Check sheet for the modelled part. Datum: model origin and axes. Units: mm. A direction names the side the tool comes from. Round coordinates to 2 decimals unless told otherwise and drop trailing zeros. Order: outer loops, then holes, each group sorted by start corner. A loop starts at its lowest first (then second) coordinate and runs counter-clockwise, first axis right, second up. Notation, with made-up numbers: (-2.75, -14.5) -> (25.25, -14.5) arc R18 ccw to (25.25, 20.5) -> close; hole circle Ø10 at (43.25, 67.5). An arc over 180 degrees is marked (long way). Answer in a Markdown table with one row per item. Add a question column.
1. Draft check along X on faces 3 (the flat face through (0, -2.8, 7)), 4 (the flat face through (0, -4.5, 7)), 5 (the cylindrical face through (-8.115, 4.199, 6.987)). Enter one of: +X half, -X half, draft (parallel to the pull), parting line (faces both ways), or undercut.
2. Sectioned sample at A-A, the plane x = -2.75. Record the boundary of the cut face in (y, z), then the cut area to 3 significant figures.
3. Sectioned sample at C-C, the plane y = -0.75. Record the boundary of the cut face in (x, z).
4. Access from +Z, -Z, +X, -X, +Y, -Y to the whole of each face (thin tool, end or side, straight path). Record for faces 1 (the flat face through (0, 0, -2)), 2 (the flat face through (0, 0, 0)).
5. Depth check by flat-ended pin: P1, Ø2, axis at x = -0.5, y = 1, coming from the +Z side. Enter the tip coordinate at first touch or a pass-through.
6. Material ranges on L1, parallel to X at y = -1.5, z = 14.25; L2, parallel to Y at x = -1, z = 11.75; L3, parallel to Z at x = -6, y = 0.25, recorded low to high. Write a range as from..to.
7. Sectioned sample at B-B, the plane z = 8.75. Record the boundary of the cut face in (x, y), then the cut area to 3 significant figures.
```python
from build123d import *

# Parameters (mm, degrees)
F0_W     = 16.8
F0_H     = 9
F0_W_2   = 13.4
F0_H_2   = 5.6
F1_DEPTH = 15.2
F2_DEPTH = 2
F3_R     = 1
F4_SIZE  = 1


with BuildPart() as f1:
    # F0 (on Top) → F1 (new body)
    with BuildSketch(Plane.XY):
        Rectangle(F0_W, F0_H)
        Rectangle(F0_W_2, F0_H_2, mode=Mode.SUBTRACT)
    extrude(amount=F1_DEPTH)

    # F0 (on Top) → F2 (join)
    with BuildSketch(Plane.XY):
        Rectangle(F0_W, F0_H)
        Rectangle(F0_W_2, F0_H_2, mode=Mode.SUBTRACT)
        Rectangle(F0_W_2, F0_H_2)
    extrude(amount=-F2_DEPTH)

    # F3
    f3_edges = [f1.edges().sort_by_distance(p)[0] for p in [
        (-8.4, 4.5, 6.6),
        (-8.4, -4.5, 6.6),
        (8.4, -4.5, 6.6),
        (8.4, 4.5, 6.6),
    ]]
    fillet(f3_edges, radius=F3_R)

    # F4
    f4_edges = [f1.edges().sort_by_distance(p)[0] for p in [
        (0, -4.5, -2),
        (-8.107107, -4.207107, -2),
        (8.107107, -4.207107, -2),
        (-8.4, 0, -2),
        (8.4, 0, -2),
        (-8.107107, 4.207107, -2),
        (8.107107, 4.207107, -2),
        (0, 4.5, -2),
    ]]
    chamfer(f4_edges, length=F4_SIZE)


solid = f1.part
```
Answer key:
| question | item | result |
|---|---|---|
| 1 | face 3 | undercut |
| 1 | face 4 | draft |
| 1 | face 5 | -X half |
| 2 | outline | (-4.5, -1) -> (-3.5, -2) -> (3.5, -2) -> (4.5, -1) -> (4.5, 15.2) -> (2.8, 15.2) -> (2.8, 0) -> (-2.8, 0) -> (-2.8, 15.2) -> (-4.5, 15.2) -> close |
| 2 | area | 68.7 mm² |
| 3 | outline | (-8.4, -1) -> (-7.4, -2) -> (7.4, -2) -> (8.4, -1) -> (8.4, 15.2) -> (6.7, 15.2) -> (6.7, 0) -> (-6.7, 0) -> (-6.7, 15.2) -> (-8.4, 15.2) -> close |
| 4 | face 1 | -Z, +X, -X, +Y, -Y |
| 4 | face 2 | +Z |
| 5 | P1 | stops at z = 0 |
| 6 | L1 | x = -8.4..-6.7, 6.7..8.4 |
| 6 | L2 | y = -4.5..-2.8, 2.8..4.5 |
| 6 | L3 | z = -2..0 |
| 7 | outline | (-8.4, -3.5) arc R1 ccw to (-7.4, -4.5) -> (7.4, -4.5) arc R1 ccw to (8.4, -3.5) -> (8.4, 3.5) arc R1 ccw to (7.4, 4.5) -> (-7.4, 4.5) arc R1 ccw to (-8.4, 3.5) -> close; hole (-6.7, -2.8) -> (6.7, -2.8) -> (6.7, 2.8) -> (-6.7, 2.8) -> close |
| 7 | area | 75.3 mm² |
